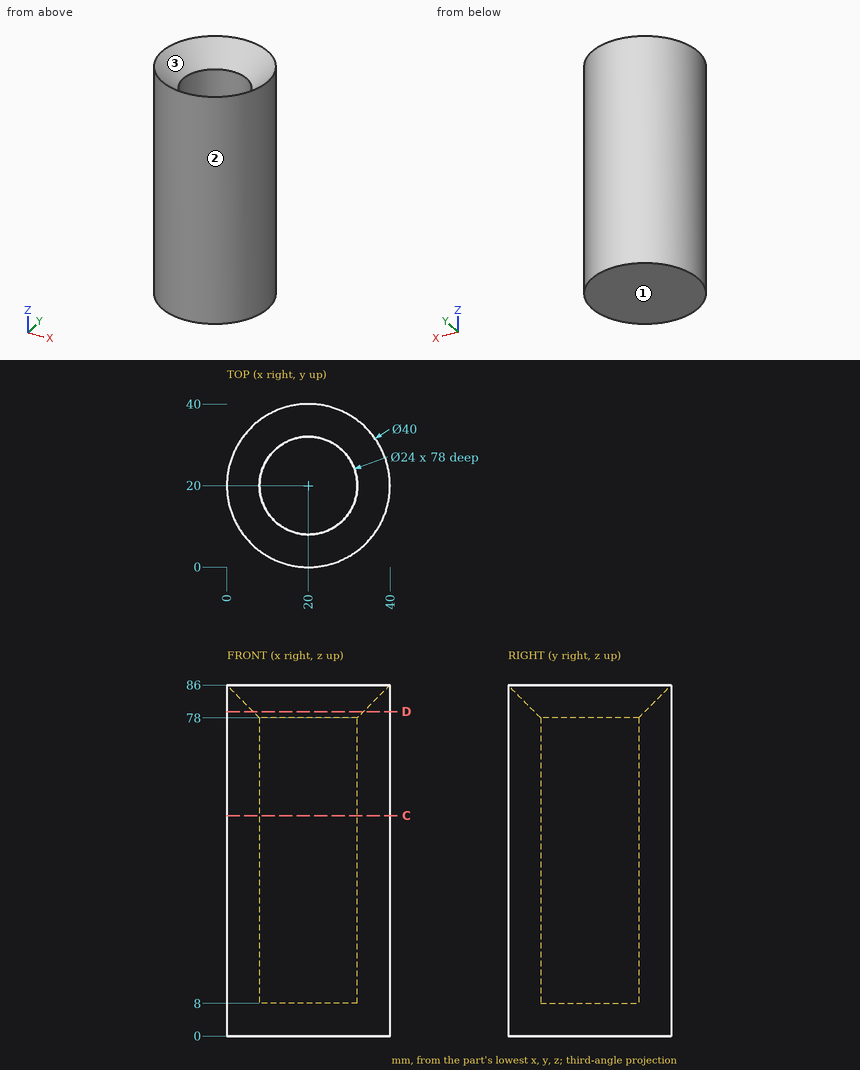
Could you check a few things on this drawing? It's one solid part, dimensions in mm from its lowest x, y, z. Coordinates: 2 decimals unless noted, no trailing zeros. Write each loop counter-clockwise with the first axis right and the second up, starting at its lowest first coordinate (ties: lowest second). Pieces come first, ordered by that corner, then holes. Notation, with made-up numbers: M -27.75,-34.5 L 31.25,-34.5 A29 cw 31.25,-7.5 Z; hole C 15,-33.75 d11. An arc over 180 degrees is marked long. Answer as CSV lines item,"result". Start each with the question number.
Q1. Suppose I cut it at C-C, the plane z = 54. List the corners of the cut face in (x, y) for me.
Q2. Will these pins go through, and if not, where does the flat tip stop? pin 1 Ø4 at (x, z) = (26, 57.5) entering from +Y; pin 2 Ø1.5 at (x, y) = (10, 23.5) entering from +Z; pin 3 Ø1.5 at (x, y) = (10.5, 29) entering from +Z.
Q3. Suppose I cut it at D-D, the plane z = 79.5. List the corners of the cut face in (x, y) for me, then the cut area to 3 significant figures.
Q4. If we mould it in two halves opening along X, with no side actions, what happens to the marked faces 1, 2 and 3? For each: pulls with the +X half, pulls with the -X half, needs draft (parallel to the pull), parting line crosses it, or undercut.
Q5. I need wall thicknesses on probe 1 along Y at (x, z) = (20, 51.5); probe 2 along X at (y, z) = (21, 47) (3 decimals); probe 3 along X at (y, z) = (10, 17). Which ranges of each line are inside material? Lowest first, please. Write a range as [from, to].
Entries:
1,outline,"C 20,20 d40; hole C 20,20 d24"
2,pin 1,"stops at y = 39.6"
2,pin 2,"stops at z = 8"
2,pin 3,"stops at z = 79.84"
3,outline,"C 20,20 d40; hole C 20,20 d27"
3,area,"684 mm²"
4,face 1,"needs draft"
4,face 2,"parting line crosses it"
4,face 3,"undercut"
5,probe 1,"y = [0, 8], [32, 40]"
5,probe 2,"x = [0.025, 8.042], [31.958, 39.975]"
5,probe 3,"x = [2.68, 13.37], [26.63, 37.32]"
